Geometry: final body of the model. Coordinates: model frame, mm. Face numbers are marked on the shaded views. Give positions to 0.01 mm unless a question says otherwise; leave off trailing zeros. Write each loop counter-clockwise with the first axis right and the second up, starting at its lowest first coordinate (ties: lowest second). Pieces come first, ordered by that corner, then holes. Notation, with made-up numbers: (50.25, -39.75) -> (102.25, -39.75) arc R27 ccw to (102.25, -8.75) -> close; hole circle Ø3 at (7, 79). An arc over 180 degrees is marked (long way). Answer as a JSON object with one key per item and string values. Group by question number.
(1) Section query A-A on x = 0. Output: boundary loops of the cut face in (y, z), plus the area to 3 significant figures.
(2) Material intervals for probe 1 along Y at (x, z) = (4.75, 6.35); probe 2 along Y at (x, z) = (0, 7.25); probe 3 along Y at (x, z) = (0, 6.35), sorted ascending.
(3) Draft query along X for the marked faces 1, 2 and 3. Return one class per face: +X half, -X half, draft (parallel to the pull), parting line (faces both ways), or undercut.
(4) Section query D-D on x = 6.25. Output: boundary loops of the cut face in (y, z), plus the area to 3 significant figures.
(5) Section query B-B on z = 6.35. Output: boundary loops of the cut face in (x, y).
(6) Contact query for a flat-ended pin moving along its axis: pin 1 Ø6 at (x, y) = (-5.5, 1.5) entering from -Z. Output: stop coordinate, or through.
(7) Section query C-C on y = 15. Output: boundary loops of the cut face in (x, z), plus the area to 3 significant figures.
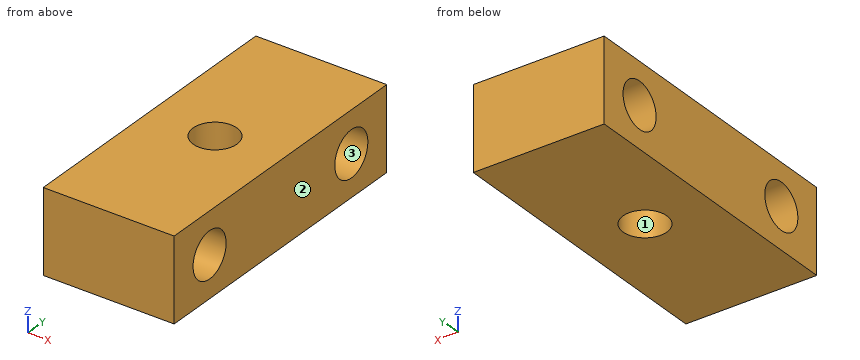
from build123d import *

# Parameters (mm, degrees)
SKETCH1_W           = 20
SKETCH1_H           = 45
BOSS_EXTRUDE1_DEPTH = 12.7
SKETCH2_R           = 3.35
CUT_EXTRUDE1_DEPTH  = 28.704512268
SKETCH3_R           = 3.5
CUT_EXTRUDE2_DEPTH  = 33.673230633


with BuildPart() as part:
    # Sketch1 → Boss-Extrude1 (new body)
    with BuildSketch(Plane.XY):
        Rectangle(SKETCH1_W, SKETCH1_H)
    extrude(amount=BOSS_EXTRUDE1_DEPTH)

    # Sketch2 → Cut-Extrude1 (cut, through all)
    with BuildSketch(Plane.XY.offset(12.7)):
        Circle(SKETCH2_R)
    extrude(amount=-CUT_EXTRUDE1_DEPTH, mode=Mode.SUBTRACT)

    # Sketch3 → Cut-Extrude2 (cut, through all)
    with BuildSketch(Plane(origin=(10, 0, 0), x_dir=(0, 0, -1), z_dir=(1, 0, 0))):
        with Locations((-6.35, 15)):
            Circle(SKETCH3_R)
        with Locations((-6.35, -15)):
            Circle(SKETCH3_R)
    extrude(amount=-CUT_EXTRUDE2_DEPTH, mode=Mode.SUBTRACT)


solid = part.part
Answer list:
{
 "1": {"outline": "(-22.5, 0) -> (-3.35, 0) -> (-3.35, 12.7) -> (-22.5, 12.7) -> close; (3.35, 0) -> (22.5, 0) -> (22.5, 12.7) -> (3.35, 12.7) -> close; hole circle Ø7 at (-15, 6.35); hole circle Ø7 at (15, 6.35)", "area": "409 mm2"},
 "2": {"probe 1": "-22.5 to -18.5, -11.5 to 11.5, 18.5 to 22.5", "probe 2": "-22.5 to -18.38, -11.62 to -3.35, 3.35 to 11.62, 18.38 to 22.5", "probe 3": "-22.5 to -18.5, -11.5 to -3.35, 3.35 to 11.5, 18.5 to 22.5"},
 "3": {"face 1": "undercut", "face 2": "+X half", "face 3": "draft"},
 "4": {"outline": "(-22.5, 0) -> (22.5, 0) -> (22.5, 12.7) -> (-22.5, 12.7) -> close; hole circle Ø7 at (-15, 6.35); hole circle Ø7 at (15, 6.35)", "area": "495 mm2"},
 "5": {"outline": "(-10, -22.5) -> (10, -22.5) -> (10, -18.5) -> (-10, -18.5) -> close; (-10, -11.5) -> (10, -11.5) -> (10, 11.5) -> (-10, 11.5) -> close; (-10, 18.5) -> (10, 18.5) -> (10, 22.5) -> (-10, 22.5) -> close; hole circle Ø6.7 at (0, 0)"},
 "6": {"pin 1": "z = 0"},
 "7": {"outline": "(-10, 0) -> (10, 0) -> (10, 2.85) -> (-10, 2.85) -> close; (-10, 9.85) -> (10, 9.85) -> (10, 12.7) -> (-10, 12.7) -> close", "area": "114 mm2"}
}
